Autodesk Inventor part; units mm, degrees
ref_plane "YZ Plane" through (0, 0, 0) normal (1, 0, 0) x (0, 1, 0)
ref_plane "XZ Plane" through (0, 0, 0) normal (0, 1, 0) x (-1, 0, 0)
ref_plane "XY Plane" through (0, 0, 0) normal (0, 0, 1) x (1, 0, 0)
sketch "Sketch1" plane through (0, 0, 0) normal (0, 0, 1) x (1, 0, 0)
  circle A0 centre (-8.485, -3.042) radius 1.1
  line L0 (-21.0171, 3.396) -> (-20.9715, -5.8039)
  line L1 (-19.9666, -6.7989) -> (3.0331, -6.6851)
  line L2 (4.0282, -5.6801) -> (3.9826, 3.5198)
  circle A1 centre (0, 0) radius 3
  circle A2 centre (-16.9998, -0.0841) radius 3
  circle A3 centre (-8.485, -3.042) radius 1
  line L3 (2.9777, 4.5148) -> (-20.022, 4.401)
  arc A4 (-20.9715, -5.8039) -> (-19.9666, -6.7989) centre (-19.9715, -5.7989) ccw
  arc A5 (3.0331, -6.6851) -> (4.0282, -5.6801) centre (3.0282, -5.6851) ccw
  arc A6 (3.9826, 3.5198) -> (2.9777, 4.5148) centre (2.9826, 3.5148) ccw
  arc A7 (-20.022, 4.401) -> (-21.0171, 3.396) centre (-20.0171, 3.401) ccw
  point P0 (0, 0)
  dimension "d0" = 2
extrude "Extrusion1" add sketch "Sketch1" against normal blind 5.1 contours A3
sketch "Sketch2" plane through (-8.485, -3.042, -5.1) normal (0, 0, -1) x (-1, 0, 0)
  circle A0 centre (0, 0) radius 1.1
  line L0 (12.5394, 7.938) -> (12.4815, -3.7618)
  line L1 (12.4815, -3.7618) -> (-12.5182, -3.6381)
  line L2 (-12.5182, -3.6381) -> (-12.4603, 8.0618)
  line L3 (-12.4603, 8.0618) -> (12.5394, 7.938)
  circle A1 centre (-8.485, 3.042) radius 3
  circle A2 centre (8.5147, 2.9579) radius 3
  line L4 (-0.0183, -3.7) -> (-0.0183, -4.9)
  circle A3 centre (0, 0) radius 4.9
  line L5 (-0.0183, -4.9) -> (-0.0183, -2.9)
  circle A4 centre (0, 0) radius 2.9
  line L6 (0, 2.9) -> (0, 3.4)
  line L7 (0, 3.4) -> (0.5456, 2.8482)
  line L8 (0, 3.4) -> (-0.5456, 2.8482)
  line L9 (-2.4042, 2.4042) -> (-1.6282, 2.3998)
  line L10 (-2.4042, 2.4042) -> (-2.3998, 1.6282)
  line L11 (-3.4, 0) -> (-2.8482, 0.5456)
  line L12 (-3.4, 0) -> (-2.8482, -0.5456)
  line L13 (-2.4042, -2.4042) -> (-2.3998, -1.6282)
  line L14 (-2.4042, -2.4042) -> (-1.6282, -2.3998)
  line L15 (0, -3.4) -> (-0.5456, -2.8482)
  line L16 (0, -3.4) -> (0.5456, -2.8482)
  line L17 (2.4042, -2.4042) -> (1.6282, -2.3998)
  line L18 (2.4042, -2.4042) -> (2.3998, -1.6282)
  line L19 (3.4, 0) -> (2.8482, -0.5456)
  line L20 (3.4, 0) -> (2.8482, 0.5456)
  line L21 (2.4042, 2.4042) -> (2.3998, 1.6282)
  line L22 (2.4042, 2.4042) -> (1.6282, 2.3998)
  line L23 (8.5147, 2.9579) -> (0, 0)
  point P0 (-8.485, 3.042)
  point P1 (2.3998, 1.6282)
  point P2 (-1.6282, 2.3998)
  point P3 (-2.3998, 1.6282)
  point P4 (-2.8482, 0.5456)
  point P5 (-2.8482, -0.5456)
  point P6 (-2.3998, -1.6282)
  point P7 (-1.6282, -2.3998)
  point P8 (-0.5456, -2.8482)
  point P9 (0.5456, -2.8482)
  point P10 (1.6282, -2.3998)
  point P11 (2.8482, -0.5456)
  point P12 (2.8482, 0.5456)
  dimension "d3" = 1.2
  dimension "d4" = 2
  dimension "d5" = 0.5
  dimension "d8" = 360
extrude "Extrusion2" add sketch "Sketch2" along normal blind 4.5 contours A0 | A4 | L20 L19 A4 | A4 L22 L21 | A4 L6 L7 | L18 L17 A4 | A4 L8 L6 | L15 A4 L5 | L5 A4 L16 L15 | A4 L10 L9 | L14 L13 A4 | A4 L12 L11
sketch "Sketch3" plane through (-8.485, -3.042, -9.6) normal (0, 0, -1) x (-1, 0, 0)
  circle A0 centre (0, 0) radius 1
  point P0 (-8.485, 3.042)
extrude "Extrusion3" add sketch "Sketch3" along normal blind 2
properties part number "kolo"
The listing builds one solid part. Answer for the finished solid, in the listing's coordinates (mm). A direction names the side the tool comes from. Give positions to 0.01 mm unless a question says otherwise; leave off trailing zeros. Loops run counter-clockwise (first coordinate to the right, second up) from the corner with the lowest first, then second, coordinate; pieces in that order, holes last. Notation, with made-up numbers: (10, 8) - (21, 8) arc R28 ccw to (21, 27) - close; hole circle Ø1 at (31.25, 47.25). An arc over 180 degrees is marked (long way). Use one line per item in the form item = value.
1. Given pin 1 Ø3 at (x, y) = (-9.5, -5.5) entering from -Z; pin 2 Ø1.5 at (x, z) = (-10, -5) entering from +Y; pin 3 Ø1.5 at (y, z) = (-5.5, -9.5) entering from +X, each flat-ended and moving along its own axis, determine where each tip first touches the part or whether it passes through.
Calculated:
pin_1 = -9.6
pin_2 = -0.25
pin_3 = -6.08
2. Section B-B on x = -8.25 is taken. Give the vertices of the cut face in (y, z), then the cut area to 3 significant figures.
Calculated:
outline = (-6.2, -9.6) - (-4.01, -9.6) - (-4.01, -11.6) - (-2.07, -11.6) - (-2.07, -9.6) - (0.12, -9.6) - (0.12, -5.1) - (-2.07, -5.1) - (-2.07, 0) - (-4.01, 0) - (-4.01, -5.1) - (-6.2, -5.1) - close
area = 42.3 mm^2
3. Find the intervals of material crossed by line 1 along Z through (x, y) = (-6, -2.75); line 2 along Y through (x, z) = (-10.25, -8.75); line 3 along X through (y, z) = (-4.5, -9.25), in increasing order. Write a range as [from, to].
Calculated:
line_1 = [-9.6, -5.1]
line_2 = [-5.44, -0.64]
line_3 = [-10.99, -5.98]
4. Section A-A on z = -6 is taken. Give the vertices of the cut face in (x, y) (3 decimals), then the cut area to 3 significant figures.
Calculated:
outline = (-11.885, -3.042) - (-11.333, -3.588) arc R2.9 ccw to (-10.885, -4.67) - (-10.889, -5.446) - (-10.113, -5.442) arc R2.9 ccw to (-9.031, -5.89) - (-8.485, -6.442) - (-7.939, -5.89) arc R2.9 ccw to (-6.857, -5.442) - (-6.081, -5.446) - (-6.085, -4.67) arc R2.9 ccw to (-5.637, -3.588) - (-5.085, -3.042) - (-5.637, -2.496) arc R2.9 ccw to (-6.085, -1.414) - (-6.081, -0.638) - (-6.857, -0.642) arc R2.9 ccw to (-7.939, -0.194) - (-8.485, 0.358) - (-9.031, -0.194) arc R2.9 ccw to (-10.113, -0.642) - (-10.889, -0.638) - (-10.885, -1.414) arc R2.9 ccw to (-11.333, -2.496) - close
area = 28.5 mm^2
5. Section C-C on y = -2.75 is taken. Give the vertices of the cut face in (x, z).
Calculated:
outline = (-11.59, -9.6) - (-9.44, -9.6) - (-9.44, -11.6) - (-7.53, -11.6) - (-7.53, -9.6) - (-5.38, -9.6) - (-5.38, -5.1) - (-7.53, -5.1) - (-7.53, 0) - (-9.44, 0) - (-9.44, -5.1) - (-11.59, -5.1) - close
6. Which of the six approach directions +Z, -Z, +X, -X, +Y, -Y give full straight-line access (tool end or side, diameter ignored) to faces 1 (the face through (-7.7, -2.2, -9.6)), 2 (the face through (-9.28, -3.65, -2.51)), 3 (the face through (-9.59, -0.36, -7.32))?
Calculated:
face_1 = -Z
face_2 = +Z
face_3 = +Z, -Z, -X, +Y
7. Section D-D on z = -2.5 is taken. Give the vertices of the cut face in (x, y) (3 decimals).
Calculated:
outline = circle Ø2 at (-8.485, -3.042)
